The drawing under review shows one solid part. Ordinate dimensions are in mm from its lowest x, y, z. Give positions to 0.01 mm unless a question says otherwise; leave off trailing zeros. Order: outer loops, then holes, each group sorted by start corner. A loop starts at its lowest first (then second) coordinate and runs counter-clockwise, first axis right, second up. Notation, with made-up numbers: (-6.5, -20) -> (29.5, -20) arc R33 ccw to (29.5, 13) -> close; hole circle Ø10 at (74, 9.25). An arc over 180 degrees is marked (long way). One line per item, written item: value.
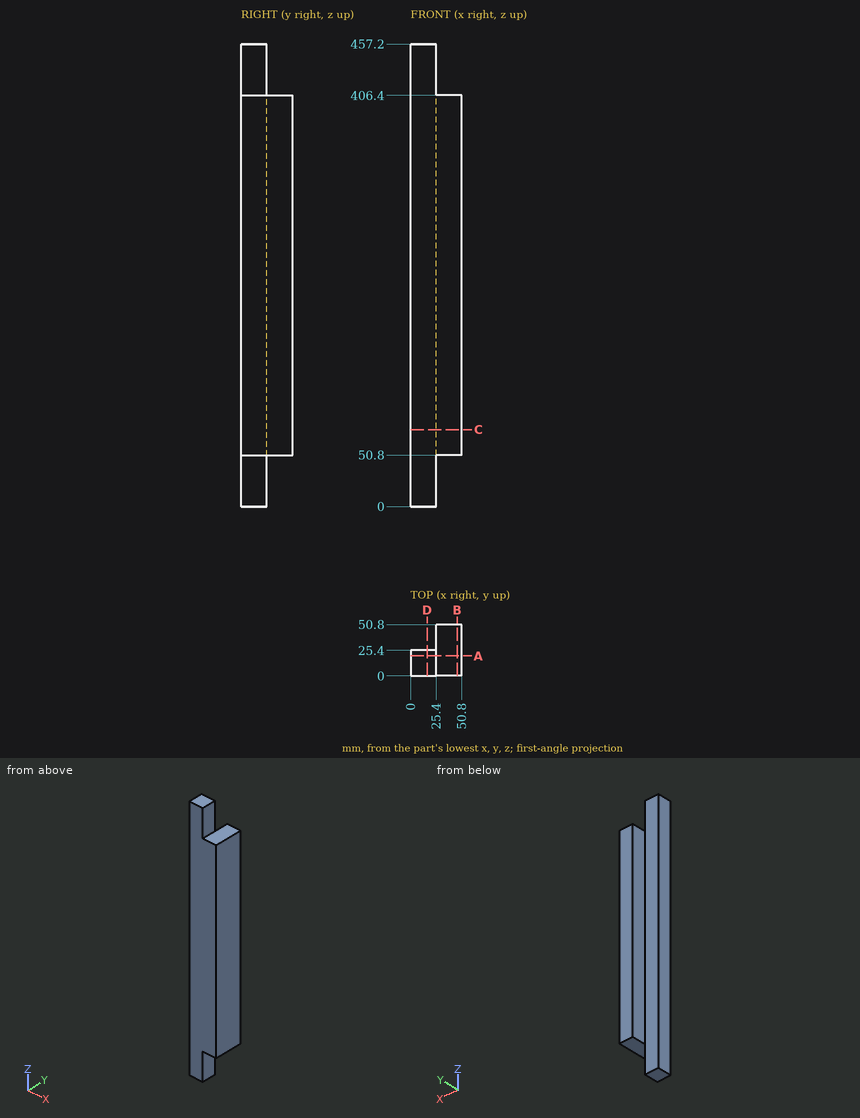
Item 1: To check wall thickness, follow line 1 along X through (y, z) = (29, 401); line 2 along Y through (x, z) = (10, 236); line 3 along Z through (x, y) = (35, 33). State the ranges of each line that lie inside material, in increasing order. Write a range as from..to.
Returned:
line 1: 25.4..50.8
line 2: 0..25.4
line 3: 50.8..406.4
Item 2: Add section D-D on x = 16.5. Give the boundary of the cut face in (y, z).
Returned:
outline: (0, 0) -> (25.4, 0) -> (25.4, 457.2) -> (0, 457.2) -> close
Item 3: Add section C-C on z = 76. Give the boundary of the cut face in (x, y), plus the area to 3 significant figures.
Returned:
outline: (0, 0) -> (50.8, 0) -> (50.8, 50.8) -> (25.4, 50.8) -> (25.4, 25.4) -> (0, 25.4) -> close
area: 1,940 mm²
Item 4: Add section A-A on y = 20. Give the boundary of the cut face in (x, z), plus the area to 3 significant figures.
Returned:
outline: (0, 0) -> (25.4, 0) -> (25.4, 50.8) -> (50.8, 50.8) -> (50.8, 406.4) -> (25.4, 406.4) -> (25.4, 457.2) -> (0, 457.2) -> close
area: 20,600 mm²
Item 5: Add section B-B on x = 46. Give the boundary of the cut face in (y, z), plus the area to 3 significant figures.
Returned:
outline: (0, 50.8) -> (50.8, 50.8) -> (50.8, 406.4) -> (0, 406.4) -> close
area: 18,100 mm²
Item 6: Clearance check with flat-ended pins moving along their axes: P1, Ø7.5, axis at y = 12, z = 428, coming from the +X side; P2, Ø1, axis at x = 22, z = 275.5, coming from the +Y side; P3, Ø12, axis at x = 27, y = 38, coming from the +Z side; P4, Ø3, axis at x = 19.5, y = 23.5, coming from the -Z side. State where each tip first meets the part, or that it passes through.
Returned:
P1: x = 25.4
P2: y = 25.4
P3: z = 406.4
P4: z = 0
